Read the model definition and answer for the solid it produces. Units are mm, in the model's axes. Give positions to 0.01 mm unless a question says otherwise; leave off trailing zeros. Order: outer loops, then holes, each group sorted by start corner. A loop starts at its lowest first (then second) coordinate and runs counter-clockwise, first axis right, second up. Notation, with made-up numbers: (47.25, 31.25) -> (52.25, 31.25) arc R27 ccw to (52.25, 69.25) -> close; hole circle Ø9 at (14.5, 88). An arc over 180 degrees is marked (long way). Use one line per item in the form item = value.
```python
from build123d import *

# Parameters (mm, degrees)
SKETCH1_R           = 67.15
BOSS_EXTRUDE1_DEPTH = 10
FILLET1_R           = 8
CUT_EXTRUDE3_REACH  = 97.49
SKETCH4_R           = 1.25


with BuildPart() as part:
    # Sketch1 → Boss-Extrude1 (new body)
    with BuildSketch(Plane(origin=(0, 0, 0), x_dir=(1, 0, 0), z_dir=(0, 1, 0))):
        with Locations(Location((0, 0, 0), (0, 0, 270))):
            Circle(SKETCH1_R)
    extrude(amount=BOSS_EXTRUDE1_DEPTH)

    # Fillet1
    fillet1_edges = [part.edges().sort_by_distance(p)[0] for p in [
        (0, 10, -67.15),
    ]]
    fillet(fillet1_edges, radius=FILLET1_R)

    # Sketch4 → Cut-Extrude3 (cut, up to next)
    with BuildSketch(Plane(origin=(0, 10, 0), x_dir=(1, 0, 0), z_dir=(0, 1, 0)), mode=Mode.PRIVATE) as cut_extrude3_sk1:
        with Locations(Location((0, 0, 0), (0, 0, 270))):
            Circle(SKETCH4_R)
    cut_extrude3_tool1 = extrude(cut_extrude3_sk1.sketch, amount=-CUT_EXTRUDE3_REACH, mode=Mode.PRIVATE) & part.part
    add(cut_extrude3_tool1.solids().sort_by_distance((0, 10, 0))[0], mode=Mode.SUBTRACT)


solid = part.part
```
Item 1: Straight lines are drawn through the part: L1, parallel to X at y = 5, z = 0; L2, parallel to Z at x = 55, y = 6.5; L3, parallel to X at y = 7.75, z = 40.5. For each, find the intervals that lie inside material, in ascending order. Write a range as from..to.
Checks:
L1 = -66.57..-1.25, 1.25..66.57
L2 = -36.05..36.05
L3 = -50.47..50.47
Item 2: The part is cut by section A-A on y = 6.5. Give the vertices of the cut face in (x, z).
Checks:
outline = circle Ø131.53 at (0, 0); hole circle Ø2.5 at (0, 0)
Item 3: Given pin 1 Ø2 at (x, y) = (43.5, 2) entering from +Z; pin 2 Ø2 at (x, z) = (38.5, 24) entering from -Y; pin 3 Ø6 at (y, z) = (9, -36.5) entering from -X; pin 4 Ø6 at (y, z) = (6, 35.5) entering from +X, each flat-ended and moving along its own axis, determine where each tip first touches the part or whether it passes through.
Checks:
pin_1 = 51.99
pin_2 = 0
pin_3 = -55.78
pin_4 = 58.08
